Model file for the job. Use its own axes, mm. A direction names the side the tool comes from. Give positions to 0.01 mm unless a question says otherwise; leave off trailing zeros. Order: outer loops, then holes, each group sorted by start corner. A loop starts at its lowest first (then second) coordinate and runs counter-clockwise, first axis right, second up. Notation, with made-up numbers: (64.5, 65) - (121.5, 65) arc R17 ccw to (121.5, 72) - close; hole circle Ø10 at (30.5, -4.75). An arc over 180 degrees is marked (long way). Use CSV: the item, a comma, the result in double quotes. Start each with the question number.
(1) Band-saw the part on A-A, the plane x = 28. Give the cut face in (y, z).
(2) Tool access for faces 5 (the cylindrical face through (-25.824, -3.131, -50.983)), 6 (the cylindrical face through (-11.766, -9.481, 0.535)): list every direction of +Z, -Z, +X, -X, +Y, -Y with a clear straight run to the whole face (end or side of a thin tool).
(3) Band-saw the part on D-D, the plane z = 29. Give the cut face in (x, y), then the cut area to 3 significant figures.
(4) Band-saw the part on C-C, the plane x = 0. Give the cut face in (y, z).
(5) Band-saw the part on B-B, the plane y = -9. Give the cut face in (x, z) (1 decimal), then the cut area to 3 significant figures.
(6) Pull direction X, two halves, no side cores. Call faces 1 (the cylindrical face through (-13.77, -3.13, -61.99)), 2 (the cylindrical face through (10.29, -9.48, -5.73)), 3 (the flat face through (-1, 0, 1)), 4 (the flat face through (25.8, -3.1, -22.3)): +X half, -X half, draft (parallel to the pull), parting line (faces both ways), or undercut.
(7) Probe L1, parallel to Z at x = 39, y = -2.5; L2, parallel to Z at x = -23, y = -2.75; L3, parallel to X at y = -2, z = -51.5. List the from-to ranges inside material, lowest first.
(8) Drop flat-ended pins along their axis: pin 1 Ø1.9 at (y, z) = (-3.5, -27) entering from +X; pin 2 Ø3 at (y, z) = (-2.5, 33) entering from +X; pin 3 Ø8 at (x, y) = (-33, -2.5) entering from +Z. Give the stop position or say it passes through.
from build123d import *

# Parameters (mm, degrees)
F0_R     = 63.5
F1_DEPTH = 6.35
F0_R_2   = 5.092997
F2_DEPTH = 12.7
F3_DEPTH = 19.05


with BuildPart() as f1:
    # F0 (on Front) → F1 (new body)
    with BuildSketch(Plane.XZ):
        Circle(F0_R)
        with BuildLine():
            ThreePointArc((57.122257, 1.780511), (57.143064, 0.890363), (57.15, 0))
            ThreePointArc((57.15, 0), (57.135905, -1.269183), (57.093628, -2.537739))
            ThreePointArc((57.093628, -2.537739), (54.98137, -15.593956), (49.924429, -27.814994))
            ThreePointArc((49.924429, -27.814994), (47.213271, -32.202943), (44.117535, -36.328579))
            ThreePointArc((44.117535, -36.328579), (25.871512, -50.958683), (3.292949, -57.055052))
            ThreePointArc((3.292949, -57.055052), (0.552387, -57.14733), (-2.189447, -57.108045))
            ThreePointArc((-2.189447, -57.108045), (-26.134958, -50.824074), (-45.176341, -35.003153))
            ThreePointArc((-45.176341, -35.003153), (-48.893175, -29.5902), (-51.964588, -23.786636))
            ThreePointArc((-51.964588, -23.786636), (-55.608023, -13.185989), (-57.112206, -2.078074))
            ThreePointArc((-57.112206, -2.078074), (-57.143101, 0.887966), (-57.020063, 3.851614))
            ThreePointArc((-57.020063, 3.851614), (-54.031986, 18.618995), (-47.288543, 32.092307))
            ThreePointArc((-47.288543, 32.092307), (-43.8631, 36.635378), (-40.002895, 40.815327))
            ThreePointArc((-40.002895, 40.815327), (-24.384219, 51.686868), (-6.061928, 56.827595))
            ThreePointArc((-6.061928, 56.827595), (-0.991719, 57.141395), (4.086326, 57.003723))
            ThreePointArc((4.086326, 57.003723), (20.760172, 53.246012), (35.57713, 44.725723))
            ThreePointArc((35.57713, 44.725723), (39.918168, 40.898195), (43.84984, 36.651249))
            ThreePointArc((43.84984, 36.651249), (53.41192, 20.329518), (57.122257, 1.780511))
        make_face(mode=Mode.SUBTRACT)
        with BuildLine():
            Line((-7.523903, 9.061736), (-40.002895, 40.815327))
            ThreePointArc((-40.002895, 40.815327), (-43.8631, 36.635378), (-47.288543, 32.092307))
            Line((-47.288543, 32.092307), (-11.370419, 3.072091))
            ThreePointArc((-11.370419, 3.072091), (-9.91049, 6.364461), (-7.523903, 9.061736))
        make_face()
        with BuildLine():
            Line((-11.615889, 1.948155), (-57.020063, 3.851614))
            ThreePointArc((-57.020063, 3.851614), (-57.143101, 0.887966), (-57.112206, -2.078074))
            Line((-57.112206, -2.078074), (-11.741675, -0.925877))
            ThreePointArc((-11.741675, -0.925877), (-11.766858, 0.514994), (-11.615889, 1.948155))
        make_face()
        with BuildLine():
            ThreePointArc((-51.964588, -23.786636), (-48.893175, -29.5902), (-45.176341, -35.003153))
            Line((-45.176341, -35.003153), (-7.989839, -8.653707))
            ThreePointArc((-7.989839, -8.653707), (-10.319767, -5.676847), (-11.586634, -2.115202))
            Line((-11.586634, -2.115202), (-51.964588, -23.786636))
        make_face()
        with BuildLine():
            ThreePointArc((44.117535, -36.328579), (47.213271, -32.202943), (49.924429, -27.814994))
            Line((49.924429, -27.814994), (11.586634, -2.115202))
            ThreePointArc((11.586634, -2.115202), (10.317636, -5.680719), (7.983341, -8.659702))
            Line((7.983341, -8.659702), (44.117535, -36.328579))
        make_face()
        with BuildLine():
            Line((11.481925, 2.6248), (43.84984, 36.651249))
            ThreePointArc((43.84984, 36.651249), (39.918168, 40.898195), (35.57713, 44.725723))
            Line((35.57713, 44.725723), (6.470598, 9.841521))
            ThreePointArc((6.470598, 9.841521), (9.674375, 6.717935), (11.481925, 2.6248))
        make_face()
        with BuildLine():
            Line((4.086326, 11.046543), (4.086326, 57.003723))
            ThreePointArc((4.086326, 57.003723), (-0.991719, 57.141395), (-6.061928, 56.827595))
            Line((-6.061928, 56.827595), (-3.825, 11.139728))
            ThreePointArc((-3.825, 11.139728), (0.138722, 11.777306), (4.086326, 11.046543))
        make_face()
        with BuildLine():
            ThreePointArc((57.093628, -2.537739), (57.135905, -1.269183), (57.15, 0))
            ThreePointArc((57.15, 0), (57.143064, 0.890363), (57.122257, 1.780511))
            Line((57.122257, 1.780511), (11.642764, 1.780511))
            ThreePointArc((11.642764, 1.780511), (11.744234, 0.892824), (11.778123, 0))
            ThreePointArc((11.778123, 0), (11.769223, -0.457783), (11.742537, -0.914875))
            Line((11.742537, -0.914875), (57.093628, -2.537739))
        make_face()
        with BuildLine():
            ThreePointArc((-2.189447, -57.108045), (0.552387, -57.14733), (3.292949, -57.055052))
            Line((3.292949, -57.055052), (3.292949, -11.308433))
            ThreePointArc((3.292949, -11.308433), (0.567368, -11.764449), (-2.189447, -11.572835))
            Line((-2.189447, -11.572835), (-2.189447, -57.108045))
        make_face()
    extrude(amount=F1_DEPTH)

    # F0 (on Front) → F2 (join)
    with BuildSketch(Plane.XZ):
        with BuildLine():
            ThreePointArc((11.778123, 0), (11.744234, 0.892824), (11.642764, 1.780511))
            ThreePointArc((11.642764, 1.780511), (11.570048, 2.204123), (11.481925, 2.6248))
            ThreePointArc((11.481925, 2.6248), (9.674375, 6.717935), (6.470598, 9.841521))
            ThreePointArc((6.470598, 9.841521), (5.312737, 10.51185), (4.086326, 11.046543))
            ThreePointArc((4.086326, 11.046543), (0.138722, 11.777306), (-3.825, 11.139728))
            ThreePointArc((-3.825, 11.139728), (-5.768788, 10.268654), (-7.523903, 9.061736))
            ThreePointArc((-7.523903, 9.061736), (-9.91049, 6.364461), (-11.370419, 3.072091))
            ThreePointArc((-11.370419, 3.072091), (-11.506885, 2.513122), (-11.615889, 1.948155))
            ThreePointArc((-11.615889, 1.948155), (-11.766858, 0.514994), (-11.741675, -0.925877))
            ThreePointArc((-11.741675, -0.925877), (-11.679303, -1.522514), (-11.586634, -2.115202))
            ThreePointArc((-11.586634, -2.115202), (-10.319767, -5.676847), (-7.989839, -8.653707))
            ThreePointArc((-7.989839, -8.653707), (-5.294789, -10.520902), (-2.189447, -11.572835))
            ThreePointArc((-2.189447, -11.572835), (0.567368, -11.764449), (3.292949, -11.308433))
            ThreePointArc((3.292949, -11.308433), (5.7916, -10.255806), (7.983341, -8.659702))
            ThreePointArc((7.983341, -8.659702), (10.317636, -5.680719), (11.586634, -2.115202))
            ThreePointArc((11.586634, -2.115202), (11.680015, -1.517042), (11.742537, -0.914875))
            ThreePointArc((11.742537, -0.914875), (11.769223, -0.457783), (11.778123, 0))
        make_face()
        Circle(F0_R_2, mode=Mode.SUBTRACT)
    extrude(amount=F2_DEPTH)

    # F0 (on Front) → F3 (join)
    with BuildSketch(Plane.XZ):
        Circle(F0_R_2)
    extrude(amount=F3_DEPTH)


solid = f1.part
Answer block:
1,outline,"(-6.35, -56.99) - (0, -56.99) - (0, -49.82) - (-6.35, -49.82) - close; (-6.35, -23.99) - (0, -23.99) - (0, -13.12) - (-6.35, -13.12) - close; (-6.35, -1.5) - (0, -1.5) - (0, 1.78) - (-6.35, 1.78) - close; (-6.35, 19.99) - (0, 19.99) - (0, 35.64) - (-6.35, 35.64) - close; (-6.35, 49.82) - (0, 49.82) - (0, 56.99) - (-6.35, 56.99) - close"
2,face 5,"+Y, -Y"
2,face 6,"-X, -Y"
3,outline,"(-56.49, -6.35) - (-49.25, -6.35) - (-49.25, 0) - (-56.49, 0) - close; (-43.46, -6.35) - (-27.92, -6.35) - (-27.92, 0) - (-43.46, 0) - close; (-4.7, -6.35) - (4.09, -6.35) - (4.09, 0) - (-4.7, 0) - close; (22.46, -6.35) - (36.57, -6.35) - (36.57, 0) - (22.46, 0) - close; (49.25, -6.35) - (56.49, -6.35) - (56.49, 0) - (49.25, 0) - close"
3,area,"336 mm2"
4,outline,"(-19.05, -5.09) - (-12.7, -5.09) - (-12.7, -11.78) - (-6.35, -11.78) - (-6.35, -63.5) - (0, -63.5) - (0, 63.5) - (-6.35, 63.5) - (-6.35, 11.78) - (-12.7, 11.78) - (-12.7, 5.09) - (-19.05, 5.09) - close"
5,outline,"(-11.7, -0.9) arc R11.8 ccw to (-11.6, -2.1) arc R11.8 ccw to (-8, -8.7) arc R11.8 ccw to (-2.2, -11.6) arc R11.8 ccw to (3.3, -11.3) arc R11.8 ccw to (8, -8.7) arc R11.8 ccw to (11.6, -2.1) arc R11.8 ccw to (11.7, -0.9) arc R11.8 ccw to (11.8, 0) arc R11.8 ccw to (11.6, 1.8) arc R11.8 ccw to (11.5, 2.6) arc R11.8 ccw to (6.5, 9.8) arc R11.8 ccw to (4.1, 11) arc R11.8 ccw to (-3.8, 11.1) arc R11.8 ccw to (-7.5, 9.1) arc R11.8 ccw to (-11.4, 3.1) arc R11.8 ccw to (-11.6, 1.9) arc R11.8 ccw to start"
5,area,"436 mm2"
6,face 1,"parting line"
6,face 2,"+X half"
6,face 3,"draft"
6,face 4,"undercut"
7,L1,"z = -50.11 to -41.77, -32.41 to -20.49, -1.89 to 1.78, 31.55 to 50.11"
7,L2,"z = -59.19 to -52.32, -19.29 to -8.24, -1.21 to 2.43, 12.47 to 24.19, 52.32 to 59.19"
7,L3,"x = -37.15 to -24.78, -2.19 to 3.29, 24.78 to 37.15"
8,pin 1,"stops at x = 57.91"
8,pin 2,"stops at x = 55.14"
8,pin 3,"stops at z = 56.49"
